CAD build for the part. Positions are in the model's coordinates, mm. A direction names the side the tool comes from. Coordinates: 2 decimals unless noted, no trailing zeros. Order: outer loops, then holes, each group sorted by start corner. A loop starts at its lowest first (then second) coordinate and runs counter-clockwise, first axis right, second up.
from build123d import *

# Parameters (mm, degrees)
SKETCH1_R           = 69.85
BOSS_EXTRUDE1_DEPTH = 3.175
SKETCH2_R           = 6.604
SKETCH2_R_2         = 3.937
SKETCH2_R_3         = 3.556
SKETCH2_R_4         = 10.668
CUT_EXTRUDE1_DEPTH  = 3.175
SKETCH3_W           = 3.81
SKETCH3_H           = 15.24
BOSS_EXTRUDE2_DEPTH = 8.382
SKETCH3_4_W         = 2.54
SKETCH3_4_H         = 3.81
SKETCH3_4_W_2       = 3.81
SKETCH3_4_H_2       = 2.54
CUT_EXTRUDE2_DEPTH  = 8.382
SKETCH4_W           = 3.81
SKETCH4_H           = 15.24
BOSS_EXTRUDE4_DEPTH = 8.382
BOSS_EXTRUDE5_DEPTH = 19.05
SKETCH6_R           = 8.128
CUT_EXTRUDE3_DEPTH  = 19.05
SKETCH7_R           = 8.128
CUT_EXTRUDE4_DEPTH  = 19.05


with BuildPart() as part:
    # Sketch1 → Boss-Extrude1 (new body)
    with BuildSketch(Plane(origin=(0, 0, 0), x_dir=(1, 0, 0), z_dir=(0, 1, 0))):
        with Locations(Location((0, 0, 0), (0, 0, 270))):
            Circle(SKETCH1_R)
    extrude(amount=BOSS_EXTRUDE1_DEPTH)

    # Sketch2 → Cut-Extrude1 (cut)
    with BuildSketch(Plane(origin=(0, 3.175, 0), x_dir=(1, 0, 0), z_dir=(0, 1, 0))):
        with Locations(Location((-53.975, 0, 0), (0, 0, 270))):
            Circle(SKETCH2_R)
        with Locations(Location((53.975, 0, 0), (0, 0, 270))):
            Circle(SKETCH2_R)
        with Locations(Location((-51.795490029, -24.152633658, 0), (0, 0, 270))):
            Circle(SKETCH2_R_2)
        with Locations(Location((51.795490029, 24.152633658, 0), (0, 0, 270))):
            Circle(SKETCH2_R_3)
        with Locations(Location((50.64447914, -23.615908466, 0), (0, 0, 270))):
            Circle(SKETCH2_R_4)
        with Locations(Location((-50.64447914, 23.615908466, 0), (0, 0, 270))):
            Circle(SKETCH2_R_4)
    extrude(amount=-CUT_EXTRUDE1_DEPTH, mode=Mode.SUBTRACT)

    # Sketch3 → Boss-Extrude2 (add)
    with BuildSketch(Plane(origin=(0, 3.175, 0), x_dir=(1, 0, 0), z_dir=(0, 1, 0))):
        with Locations((-30.607, 49.276)):
            Rectangle(SKETCH3_W, SKETCH3_H)
    extrude(amount=BOSS_EXTRUDE2_DEPTH)

    # Sketch3<4> → Cut-Extrude2 (cut)
    with BuildSketch(Plane(origin=(0, 3.175, 0), x_dir=(1, 0, 0), z_dir=(0, 1, 0))):
        with Locations((-39.37, 0)):
            Rectangle(SKETCH3_4_W, SKETCH3_4_H)
        with Locations((-39.37, -30.48)):
            Rectangle(SKETCH3_4_W, SKETCH3_4_H)
        with Locations((39.37, -30.48)):
            Rectangle(SKETCH3_4_W, SKETCH3_4_H)
        with Locations((39.37, 0)):
            Rectangle(SKETCH3_4_W, SKETCH3_4_H)
        with Locations((0, 20.32)):
            Rectangle(SKETCH3_4_W_2, SKETCH3_4_H_2)
        with Locations((0, -50.8)):
            Rectangle(SKETCH3_4_W_2, SKETCH3_4_H_2)
        with Locations((-16.51, 57.15)):
            Rectangle(SKETCH3_4_W_2, SKETCH3_4_H_2)
        with Locations((16.51, 57.15)):
            Rectangle(SKETCH3_4_W_2, SKETCH3_4_H_2)
        with Locations((16.51, 39.37)):
            Rectangle(SKETCH3_4_W_2, SKETCH3_4_H_2)
        with Locations((-16.51, 39.37)):
            Rectangle(SKETCH3_4_W_2, SKETCH3_4_H_2)
    extrude(amount=-CUT_EXTRUDE2_DEPTH, mode=Mode.SUBTRACT)

    # Sketch4 → Boss-Extrude4 (add)
    with BuildSketch(Plane(origin=(0, 3.175, 0), x_dir=(1, 0, 0), z_dir=(0, 1, 0))):
        with Locations((30.607, 49.276)):
            Rectangle(SKETCH4_W, SKETCH4_H)
    extrude(amount=BOSS_EXTRUDE4_DEPTH)

    # Sketch5 → Boss-Extrude5 (add)
    with BuildSketch(Plane(origin=(0, 3.175, 0), x_dir=(1, 0, 0), z_dir=(0, 1, 0))):
        with BuildLine():
            Line((-22.060225105, 66.27494978), (-21.331257294, 64.841108186))
            ThreePointArc((-21.331257294, 64.841108186), (2.077551681, 68.228114642), (25.236913051, 63.423103584))
            Line((25.236913051, 63.423103584), (25.974086879, 64.841108186))
            ThreePointArc((25.974086879, 64.841108186), (2.084119461, 69.818901066), (-22.060225105, 66.27494978))
        make_face()
        with BuildLine():
            Line((-22.060225105, -66.27494978), (-20.764940728, -65.218037135))
            ThreePointArc((-20.764940728, -65.218037135), (1.754255855, -68.421471174), (24.07970803, -64.068266657))
            Line((24.07970803, -64.068266657), (25.012599469, -65.218037135))
            ThreePointArc((25.012599469, -65.218037135), (1.567926874, -69.832400111), (-22.060225105, -66.27494978))
        make_face()
    extrude(amount=BOSS_EXTRUDE5_DEPTH)

    # Sketch6 → Cut-Extrude3 (cut)
    with BuildSketch(Plane(origin=(2.084119461, 22.225, -69.818901066), x_dir=(-0.9995547754627743, 0, -0.02983707173237782), z_dir=(0.029837071732377825, 0, -0.9995547754627744))):
        with Locations((0, -9.386828468)):
            Circle(SKETCH6_R)
    extrude(amount=-CUT_EXTRUDE3_DEPTH, mode=Mode.SUBTRACT)

    # Sketch7 → Cut-Extrude4 (cut)
    with BuildSketch(Plane(origin=(1.567926874, 22.225, 69.832400111), x_dir=(0.9997480330908115, 0, -0.022447056177901516), z_dir=(0.022447056177901513, 0, 0.9997480330908114))):
        with Locations((0, -10.16)):
            Circle(SKETCH7_R)
    extrude(amount=-CUT_EXTRUDE4_DEPTH, mode=Mode.SUBTRACT)


solid = part.part
1) Slice it at C-C (y = 16.75). List the corners of the cut face in (x, z), plus the area to 3 significant figures.
2) Slice it at B-B (x = 16.5). List the corners of the cut face in (y, z) (1 decimal), plus the area to 3 significant figures.
3) Pin check, flat tips, straight feed: P1, Ø0.8, axis at y = 1, z = -20.5, coming from the -X side; P2, Ø1.5, axis at x = 47.5, z = 6, coming from the +Y side (3 decimals); P3, Ø3, axis at x = 31, z = -52.5, coming from the +Y side. Stop position of each tip, or through.
4) Slice it at A-A (z = 0). List the corners of the cut face in (x, y) (3 decimals), plus the area to 3 significant figures.
5) Slice it at D-D (x = 0). Give the number of separate pieces and of enclosed holes in the cut face, plus the area to 3 significant figures.
6) Drill centre lines: probe 1 along X at (y, z) = (4.25, -55.5); probe 2 along Y at (x, z) = (20.5, -31) (3 decimals); probe 3 along Z at (x, y) = (-5.5, 6). Where is each one in solid material? Low to high.
7) Two-plate mould, pull along X, no slides. Class faces 1 (the cylindrical face through (48.64, 1.61, -22.51)), 2 (the flat face through (31, 7, -56.896)), 3 (the flat face through (-32.512, 7, -49)): released by +X, released by -X, zero draft, split by the parting line, or undercut.
8) Which spindle directions (+Z, -Z, +X, -X, +Y, -Y) get a long thin tool onto all of the face, cutting with end or side? Do faces 4 (the flat face through (16, 2, -55.88)), 5 (the flat face through (-28.702, 7, -49)), 6 (the flat face through (-31, 7, -56.896)). Say none if no direction does.
Worked out:
1. outline: (-22.06, -66.27) arc R69.85 ccw to (-5.05, -69.67) - (-5.1, -68.07) arc R68.26 cw to (-21.33, -64.84) - close; (-22.06, 66.27) - (-20.76, 65.22) arc R68.44 cw to (-5.11, 68.25) - (-5.08, 69.67) arc R69.85 ccw to start; (8.17, 67.95) arc R68.44 cw to (24.08, 64.07) - (25.01, 65.22) arc R69.85 ccw to (8.2, 69.37) - close; (9.15, -67.64) - (9.19, -69.24) arc R69.85 ccw to (25.97, -64.84) - (25.24, -63.42) arc R68.26 cw to start
1. area: 101 mm2
2. outline: (0, -67.9) - (22.2, -67.9) - (22.2, -66.2) - (3.2, -66.2) - (3.2, -58.4) - (0, -58.4) - close; (0, -55.9) - (3.2, -55.9) - (3.2, -40.6) - (0, -40.6) - close; (0, -38.1) - (3.2, -38.1) - (3.2, 66.4) - (22.2, 66.4) - (22.2, 67.9) - (0, 67.9) - close
2. area: 474 mm2
3. P1: stops at x = -66.9
3. P2: stops at y = 3.175
3. P3: stops at y = 11.56
4. outline: (-69.85, 0) - (-60.579, 0) - (-60.579, 3.175) - (-69.85, 3.175) - close; (-47.371, 0) - (-40.64, 0) - (-40.64, 3.175) - (-47.371, 3.175) - close; (-38.1, 0) - (38.1, 0) - (38.1, 3.175) - (-38.1, 3.175) - close; (40.64, 0) - (47.371, 0) - (47.371, 3.175) - (40.64, 3.175) - close; (60.579, 0) - (69.85, 0) - (69.85, 3.175) - (60.579, 3.175) - close
4. area: 344 mm2
5. separate pieces: 5
5. enclosed holes: 0
5. area: 437 mm2
6. probe 1: x = -32.51 to -28.7, 28.7 to 32.51
6. probe 2: y = 0 to 3.175
6. probe 3: z = -69.63 to -68.04, 68.22 to 69.63
7. face 1: undercut
7. face 2: zero draft
7. face 3: released by -X
8. face 4: +Y, -Y
8. face 5: +Z, -Z, +Y
8. face 6: -Z, +X, -X, +Y
